Read the model definition and answer for the solid it produces. Units are mm, in the model's axes. A direction names the side the tool comes from. Coordinates: 2 decimals unless noted, no trailing zeros. Loops run counter-clockwise (first coordinate to the right, second up) from the corner with the lowest first, then second, coordinate; pieces in that order, holes last. Notation, with made-up numbers: (43, 58) -> (85, 58) arc R27 cw to (85, 82) -> close; hole circle Ø1 at (12.5, -20). An arc over 180 degrees is marked (long way). Answer as a JSON object with one key per item and string values. Group by question number.
1) Flat-ended cylindrical pins translate along their axes: P1, Ø12, axis at y = 9, z = -20.5, coming from the -X side; P2, Ø1, axis at x = 7.5, z = -8.5, coming from the -Y side; P3, Ø10, axis at y = 23, z = 16, coming from the -X side. Find the tip coordinate at first contact, or state that the pin passes through.
2) Section B-B, the plane x = -11 is taken. Give the vertices of the cut face in (y, z), plus the area to 3 significant figures.
3) Consider probe 1 along Z at (x, y) = (4, 12.5); probe 2 along Y at (x, z) = (-16.5, 2); probe 3 along X at (y, z) = (6.75, -4.5). Determine where each line is inside the solid, lowest interval first. Write a range as [from, to].
4) Section D-D, the plane z = -19 is taken. Give the vertices of the cut face in (x, y).
5) Section C-C, the plane y = 9.75 is taken. Give the vertices of the cut face in (x, z).
6) Section A-A, the plane z = 0 is taken. Give the vertices of the cut face in (x, y).
7) Which of the six approach directions +Z, -Z, +X, -X, +Y, -Y give full straight-line access (tool end or side, diameter ignored) to faces 4 (the face through (0.855, 12.985, 0.327)), 5 (the face through (-12.516, 23.629, -20.95)), 6 (the face through (8.423, 7.726, 4.442))?
8) Determine the mould class of faces 1 (the face through (1, -0.254, 2)), 2 (the face through (-28.538, 13.114, -7.045)), 3 (the face through (-2, 15.932, -5)) for opening direction X: released by +X, released by -X, zero draft, split by the parting line, or undercut.
from build123d import *

# Parameters (mm, degrees)
SKETCH1_R                = 32.5
BOSS_EXTRUDE1_DEPTH      = 26.6
SKETCH2_R                = 26.4
CUT_EXTRUDE1_DEPTH       = 6.026
SKETCH5_R                = 25.9
CUT_EXTRUDE2_DEPTH       = 15.932
BOSS_EXTRUDE2_DEPTH      = 6.026
BOSS_EXTRUDE2_DEPTH_BACK = 20.828
SKETCH6_R                = 6.9
CUT_EXTRUDE3_DEPTH       = 13.462
CUT_EXTRUDE3_DEPTH_BACK  = 49.714
SKETCH7_R                = 1.83


with BuildPart() as part:
    # Sketch1 → Boss-Extrude1 (new body)
    with BuildSketch(Plane(origin=(0, 0, 0), x_dir=(1, 0, 0), z_dir=(0, 1, 0))):
        with Locations(Location((3.189451159, 0, 0), (0, 0, 270))):
            Circle(SKETCH1_R)
    extrude(amount=BOSS_EXTRUDE1_DEPTH)

    # Sketch2 → Cut-Extrude1 (cut)
    with BuildSketch(Plane(origin=(0, 26.6, 0), x_dir=(1, 0, 0), z_dir=(0, 1, 0))):
        with Locations(Location((3.547856728, 0, 0), (0, 0, 270))):
            Circle(SKETCH2_R)
    extrude(amount=-CUT_EXTRUDE1_DEPTH, mode=Mode.SUBTRACT)

    # Sketch5 → Cut-Extrude2 (cut)
    with BuildSketch(Plane.XZ):
        with Locations(Location((2.920646982, 0, 0), (0, 0, 270))):
            Circle(SKETCH5_R)
    extrude(amount=-CUT_EXTRUDE2_DEPTH, mode=Mode.SUBTRACT)

    # Sketch6 → Boss-Extrude2 (add, two sides: drawn at the far end of the back side and taken through both)
    with BuildSketch(Plane(origin=(0, 20.574, 0), x_dir=(1, 0, 0), z_dir=(0, 1, 0)).offset(-BOSS_EXTRUDE2_DEPTH_BACK)):
        with Locations(Location((2.605158488, -0.732268174, 0), (0, 0, 270))):
            Circle(SKETCH6_R)
    extrude(amount=BOSS_EXTRUDE2_DEPTH + BOSS_EXTRUDE2_DEPTH_BACK)

    # Sketch7 → Cut-Extrude3 (cut, two sides: drawn at the far end of the back side and taken through both)
    with BuildSketch(Plane(origin=(0, 26.6, 0), x_dir=(1, 0, 0), z_dir=(0, 1, 0)).offset(-CUT_EXTRUDE3_DEPTH_BACK)):
        with Locations(Location((2.641417448, -0.724168536, 0), (0, 0, 270))):
            Circle(SKETCH7_R)
    extrude(amount=CUT_EXTRUDE3_DEPTH + CUT_EXTRUDE3_DEPTH_BACK, mode=Mode.SUBTRACT)


solid = part.part
Determined:
{
 "1": {"P1": "x = -25.9", "P2": "y = 15.93", "P3": "x = -27.39"},
 "2": {"outline": "(0, -29.24) -> (26.6, -29.24) -> (26.6, -22.03) -> (20.57, -22.03) -> (20.57, 22.03) -> (26.6, 22.03) -> (26.6, 29.24) -> (0, 29.24) -> (0, 21.84) -> (15.93, 21.84) -> (15.93, -21.84) -> (0, -21.84) -> close", "area": "594 mm²"},
 "3": {"probe 1": "[-32.49, -25.88], [-6.03, -0.5], [1.95, 7.49], [25.88, 32.49]", "probe 2": "[15.93, 20.57]", "probe 3": "[-29, -22.59], [-1.89, 7.1], [28.43, 35.38]"},
 "4": {"outline": "(-23.18, 0) -> (-14.68, 0) -> (-14.68, 15.93) -> (20.52, 15.93) -> (20.52, 0) -> (29.56, 0) -> (29.56, 26.6) -> (21.88, 26.6) -> (21.88, 20.57) -> (-14.78, 20.57) -> (-14.78, 26.6) -> (-23.18, 26.6) -> close"},
 "5": {"outline": "circle Ø65 at (3.19, 0); circle Ø13.8 at (2.61, 0.73); hole circle Ø51.8 at (2.92, 0); hole circle Ø3.66 at (2.64, 0.72)"},
 "6": {"outline": "(-29.31, 0) -> (-22.98, 0) -> (-22.98, 15.93) -> (-4.26, 15.93) -> (-4.26, -0.25) -> (0.96, -0.25) -> (0.96, 26.6) -> (-4.26, 26.6) -> (-4.26, 20.57) -> (-22.85, 20.57) -> (-22.85, 26.6) -> (-29.31, 26.6) -> close; (4.32, -0.25) -> (9.47, -0.25) -> (9.47, 15.93) -> (28.82, 15.93) -> (28.82, 0) -> (35.69, 0) -> (35.69, 26.6) -> (29.95, 26.6) -> (29.95, 20.57) -> (9.47, 20.57) -> (9.47, 26.6) -> (4.32, 26.6) -> close"},
 "7": {"face 4": "+Y, -Y", "face 5": "+Y", "face 6": "-Y"},
 "8": {"face 1": "zero draft", "face 2": "split by the parting line", "face 3": "undercut"}
}
